Build history of the part. All positions in model axes, mm. Face numbers are marked on the shaded views. A direction names the side the tool comes from. Coordinates: 2 decimals unless noted, no trailing zeros. Order: outer loops, then holes, each group sorted by start corner. A loop starts at its lowest first (then second) coordinate and runs counter-clockwise, first axis right, second up. Notation, with made-up numbers: (34.25, 54) - (81.25, 54) arc R31 cw to (81.25, 90) - close; hole circle Ø11 at (59, 35.25). An arc over 180 degrees is marked (long way). One line per item, written item: value.
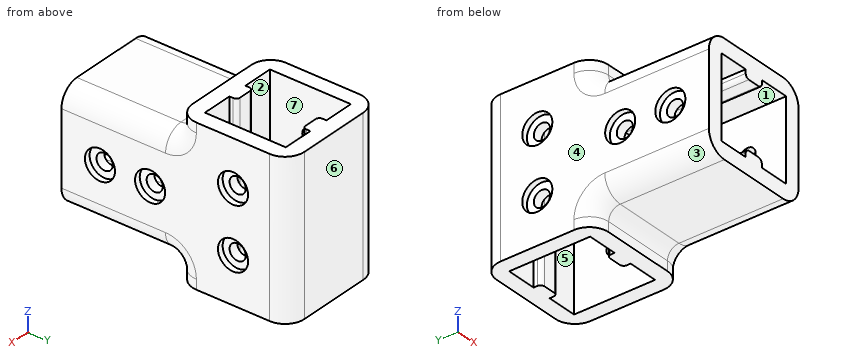
Autodesk Inventor part; units mm, degrees
ref_plane "작업 평면1" through (0, -10.5, 0) normal (1, 0, 0) x (0, 0, -1)
ref_plane "YZ Plane" through (0, 0, 0) normal (1, 0, 0) x (0, 1, 0)
ref_plane "XZ Plane" through (0, 0, 0) normal (0, 1, 0) x (-1, 0, 0)
sketch "스케치1" plane through (0, 0, 0) normal (0, 0, 1) x (1, 0, 0)
  line L0 (-10.5, -10.5) -> (10.5, -10.5)
  line L1 (10.5, -10.5) -> (10.5, 10.5)
  line L2 (10.5, 10.5) -> (-10.5, 10.5)
  line L3 (-10.5, 10.5) -> (-10.5, -10.5)
  line L4 (-10.5, -10.5) -> (10.5, 10.5) construction
  line L5 (10.5, -10.5) -> (-10.5, 10.5) construction
  line L6 (-2.6, 10.5) -> (2.6, 10.5)
  line L7 (2.6, 10.5) -> (2.6, 8.5)
  line L8 (2.6, 8.5) -> (-2.6, 8.5)
  line L9 (-2.6, 8.5) -> (-2.6, 10.5)
  line L10 (-2.6, -10.5) -> (2.6, -10.5)
  line L11 (2.6, -10.5) -> (2.6, -8.5)
  line L12 (2.6, -8.5) -> (-2.6, -8.5)
  line L13 (-2.6, -8.5) -> (-2.6, -10.5)
  line L14 (0, -20.3) -> (0, 20.3)
  line L15 (-14.5, 14.5) -> (14.5, 14.5)
  line L16 (14.5, 14.5) -> (14.5, -14.5)
  line L17 (14.5, -14.5) -> (-14.5, -14.5)
  line L18 (-14.5, -14.5) -> (-14.5, 14.5)
  point P0 (0, 0)
  dimension "d0" = 21
  dimension "d1" = 5.2
  dimension "d2" = 2
  dimension "d3" = 4
extrude "돌출1" add sketch "스케치1" along normal blind 40 contours L0 L14 L17 L18 L15 L2 L3 | L13 L12 L14 L0 | L14 L12 L11 L0 | L0 L1 L2 L14 L15 L16 L17 | L2 L14 L8 L9 | L2 L7 L8 L14
sketch "스케치2" plane through (-14.5, -14.5, 0) normal (0, -1, 0) x (1, 0, 0)
  line L0 (29, 40) -> (0, 40)
  line L1 (0, 40) -> (29, 0) construction
  line L2 (29, 0) -> (0, 0)
  line L3 (29, 40) -> (0, 0) construction
  line L4 (4, 30.5) -> (25, 30.5)
  line L5 (25, 30.5) -> (25, 9.5)
  line L6 (25, 9.5) -> (4, 9.5)
  line L7 (4, 9.5) -> (4, 30.5)
  line L8 (4, 30.5) -> (25, 9.5) construction
  line L9 (25, 30.5) -> (4, 9.5) construction
  line L10 (29, 5.5) -> (29, 34.5)
  line L11 (29, 34.5) -> (0, 34.5)
  line L12 (0, 34.5) -> (0, 5.5)
  line L13 (0, 5.5) -> (29, 5.5)
  line L14 (11.9, 28.5) -> (17.1, 28.5)
  line L15 (17.1, 28.5) -> (17.1, 30.5)
  line L16 (17.1, 30.5) -> (11.9, 30.5)
  line L17 (11.9, 30.5) -> (11.9, 28.5)
  line L18 (11.9, 28.5) -> (17.1, 30.5) construction
  line L19 (17.1, 28.5) -> (11.9, 30.5) construction
  line L20 (11.9, 9.5) -> (17.1, 9.5)
  line L21 (17.1, 9.5) -> (17.1, 11.5)
  line L22 (17.1, 11.5) -> (11.9, 11.5)
  line L23 (11.9, 11.5) -> (11.9, 9.5)
  line L24 (11.9, 9.5) -> (17.1, 11.5) construction
  line L25 (17.1, 9.5) -> (11.9, 11.5) construction
  point P0 (14.5, 0)
  point P1 (14.5, 20)
  point P2 (14.5, 29.5)
  point P3 (14.5, 10.5)
  point P4 (14.5, 29.5)
  point P5 (14.5, 20)
  point P6 (14.5, 10.5)
  point P7 (14.5, 20)
  point P8 (11.9, 30.5)
  dimension "d6" = 21
  dimension "d7" = 4
  dimension "d8" = 2
  dimension "d9" = 5.2
extrude "돌출2" add sketch "스케치2" along normal blind 30 contours L4 L15 L14 L17 | L23 L22 L21 L6 | L13 L12 L11 L10
sketch "스케치3" plane through (14.5, -14.5, 0) normal (1, 0, 0) x (0, 0, -1)
  line L0 (0, 25) -> (0, 4)
  line L1 (0, 4) -> (-40, 4)
  line L2 (-40, 25) -> (-40, 4)
  line L3 (0, 25) -> (-40, 25)
  line L4 (-9.5, 0) -> (-30.5, 0)
  line L5 (-9.5, 0) -> (-9.5, -30)
  line L6 (-30.5, -30) -> (-9.5, -30)
  line L7 (-30.5, 0) -> (-30.5, -30)
  circle A0 centre (-12, 14.5) radius 10.5 construction
  circle A1 centre (-12, 14.5) radius 2.1
  circle A2 centre (-28, 14.5) radius 2.1
  circle A3 centre (-20, -7) radius 10.5 construction
  circle A4 centre (-20, -7) radius 2.1
  circle A5 centre (-20, -20) radius 2.1
  point P0 (0, 14.5)
  dimension "d12" = 4.2
  dimension "d13" = 12
  dimension "d14" = 12
  dimension "d15" = 7
  dimension "d16" = 10
extrude "돌출3" cut sketch "스케치3" against normal through all contours A1 | A2 | A4 | A5
sketch "스케치4" plane through (14.5, -14.5, 0) normal (1, 0, 0) x (0, 0, -1)
  circle A0 centre (-28, 14.5) radius 2.1
  circle A1 centre (-12, 14.5) radius 2.1
  line L0 (0, 0) -> (0, 29)
  line L1 (0, 29) -> (-40, 29)
  line L2 (-40, 0) -> (-40, 29)
  line L3 (-34.5, 0) -> (-40, 0)
  circle A2 centre (-12, 14.5) radius 3.9
  circle A3 centre (-28, 14.5) radius 3.9
  circle A4 centre (-20, -7) radius 3.9
  circle A5 centre (-20, -20) radius 3.9
  line L4 (-34.5, 0) -> (-34.5, -30)
  line L5 (-5.5, -30) -> (-34.5, -30)
  line L6 (-5.5, 0) -> (-5.5, -30)
  line L7 (0, 0) -> (-5.5, 0)
  point P0 (0, 14.5)
  dimension "d19" = 7.8
extrude "돌출4" cut sketch "스케치4" against normal blind 1.5 contours A2 | A3 | A4 | A5
ref_plane "작업 평면1" through (0, -10.5, 0) normal (1, 0, 0) x (0, 0, -1)
mirror "미러1" about plane through (0, -10.5, 0) normal (1, 0, 0) of "돌출4"
fillet "모깎기1" radius 5 10 edges at (14.5, -14.5, 2.75) (14.5, -29.5, 5.5) (-14.5, -14.5, 2.75) (-14.5, -29.5, 5.5) (14.5, -14.5, 37.25) (-14.5, -14.5, 37.25) (-14.5, -29.5, 34.5) (14.5, -29.5, 34.5) (14.5, 14.5, 20) (-14.5, 14.5, 20)
fillet "모깎기1" radius 3 2 edges at (0, -14.5, 34.5) (0, -14.5, 5.5)
fillet "모깎기1" radius 1 8 edges at (2.6, 8.5, 20) (-2.6, 8.5, 20) (2.6, -8.5, 20) (-2.6, -8.5, 20) (2.6, -29.5, 11.5) (-2.6, -29.5, 11.5) (-2.6, -29.5, 28.5) (2.6, -29.5, 28.5)
sketch "스케치5" plane through (2.6, -14.5, 30.5) normal (0, -1, 0) x (1, 0, 0)
  line L0 (7.9, 0) -> (0, 0)
  line L1 (0, 0) -> (0, -1)
  arc A0 (-1, -2) -> (0, -1) centre (-1, -1) ccw
  line L2 (-1, -2) -> (-4.2, -2)
  arc A1 (-5.2, -1) -> (-4.2, -2) centre (-4.2, -1) ccw
  line L3 (-5.2, -1) -> (-5.2, 0)
  line L4 (-5.2, 0) -> (-13.1, 0)
  line L5 (-13.1, 0) -> (-13.1, -21)
  line L6 (-13.1, -21) -> (-5.2, -21)
  line L7 (-5.2, -21) -> (-5.2, -20)
  arc A2 (-4.2, -19) -> (-5.2, -20) centre (-4.2, -20) ccw
  line L8 (-4.2, -19) -> (-1, -19)
  arc A3 (0, -20) -> (-1, -19) centre (-1, -20) ccw
  line L9 (0, -20) -> (0, -21)
  line L10 (0, -21) -> (7.9, -21)
  line L11 (7.9, -21) -> (7.9, 0)
  line L12 (-10.6, -18.5) -> (-10.6, -2.5)
  line L13 (-10.6, -2.5) -> (-7.3623, -2.5)
  arc A4 (-7.3623, -2.5) -> (-4.2, -4.5) centre (-4.2, -1) ccw
  line L14 (-4.2, -4.5) -> (-1, -4.5)
  arc A5 (-1, -4.5) -> (2.1623, -2.5) centre (-1, -1) ccw
  line L15 (2.1623, -2.5) -> (5.4, -2.5)
  line L16 (5.4, -2.5) -> (5.4, -18.5)
  line L17 (5.4, -18.5) -> (2.1623, -18.5)
  arc A6 (2.1623, -18.5) -> (-1, -16.5) centre (-1, -20) ccw
  line L18 (-1, -16.5) -> (-4.2, -16.5)
  arc A7 (-4.2, -16.5) -> (-7.3623, -18.5) centre (-4.2, -20) ccw
  line L19 (-7.3623, -18.5) -> (-10.6, -18.5)
  point P0 (-2.6, -30.5)
  dimension "d25" = 2.5
extrude "돌출5" cut sketch "스케치5" against normal blind 2 contours L11 L10 L9 A3 L8 A2 L7 L6 L5 L4 L3 A1 L2 A0 L1 L0 | L12 L13 A4 L14 A5 L15 L16 L17 A6 L18 A7 L19
properties part number "profile_bracket"
1. Band-saw the part on B-B, the plane z = 20. Count the separate pieces of the cut face and the enclosed holes in it, and give its area (3 significant figures).
Values found:
separate pieces: 5
enclosed holes: 1
area: 518 mm2
2. 3-axis set-ups, long thin cutter, end or side, ignore diameter. For the marked faces 1, 2 and 3: which of +Z, -Z, +X, -X, +Y, -Y reach the whole face in a straight line?
Values found:
face 1: -Y
face 2: +Z, -Z
face 3: -Z, -X, -Y
3. Two-plate mould, pull along X, no slides. Class the marked faces 4, 5, 6 and 7: pulls with the +X half, pulls with the -X half, needs draft (parallel to the pull), parting line crosses it, or undercut.
Values found:
face 4: pulls with the -X half
face 5: undercut
face 6: needs draft
face 7: undercut
4. Band-saw the part on A-A, the plane y = -7. Give the cut face in (x, z).
Values found:
outline: (-14.5, 0) - (-10.5, 0) - (-10.5, 40) - (-14.5, 40) - close; (10.5, 0) - (14.5, 0) - (14.5, 40) - (10.5, 40) - close
5. Flat gauge pins, fed straight in: P1, Ø4, axis at y = -21.5, z = 20, coming from the -X side; P2, Ø5.5, axis at y = 0, z = 28, coming from the -X side; P3, Ø6, axis at y = -22.5, z = 20, coming from the +X side; P4, Ø5.5, axis at y = 0, z = 12, coming from the +X side. Where does each tip first touch, or does it go through?
Values found:
P1: passes through
P2: stops at x = -13
P3: stops at x = 14.5
P4: stops at x = 13
6. Probe line 1 along Y through (x, z) = (8.75, 28); line 2 along Z through (x, y) = (-8.5, -38); line 3 along X through (y, z) = (-3, 29.5). List the from-to ranges inside material, lowest first.
Values found:
line 1: y = -12.5 to -10.5, 10.5 to 14.5
line 2: z = 5.5 to 9.5, 30.5 to 34.5
line 3: x = -13 to -10.5, 10.5 to 13
